Here's how the part is built. I have some questions about the finished solid (model axes, mm). Round coordinates to 2 decimals unless told otherwise and drop trailing zeros. Loops run counter-clockwise (first coordinate to the right, second up) from the corner with the lowest first, then second, coordinate; pieces in that order, holes last. Notation, with made-up numbers: (55, 81) - (101, 81) arc R25 ccw to (101, 114) - close; hole circle Ø5 at (-23.75, 13). An arc over 180 degrees is marked (long way). Return JSON: item names as keys, results as strings. Group by question number.
Autodesk Inventor part; units mm, degrees
ref_plane "YZ Plane" through (0, 0, 0) normal (1, 0, 0) x (0, 1, 0)
ref_plane "XZ Plane" through (0, 0, 0) normal (0, 1, 0) x (-1, 0, 0)
ref_plane "XY Plane" through (0, 0, 0) normal (0, 0, 1) x (1, 0, 0)
sketch "Sketch1" plane through (0, 0, 0) normal (0, 1, 0) x (-1, 0, 0)
  line L0 (0, 0) -> (400, 0)
  line L1 (400, 0) -> (400, -100)
  line L2 (400, -100) -> (0, -100)
  line L3 (320, -103) -> (320, -100)
  line L4 (80, -103) -> (80, -100)
  line L5 (240, -100) -> (240, -103)
  line L6 (160, -103) -> (160, -100)
  line L7 (400, -25) -> (400, -50)
  line L8 (200, 0) -> (200, -100) construction
  line L9 (320, -103) -> (240, -103)
  line L10 (160, -103) -> (80, -103)
  line L11 (400, 0) -> (0, 0)
  line L12 (400, -100) -> (400, 0)
  line L13 (400, -25) -> (400, -50)
  line L14 (400, 0) -> (400, -100)
  line L15 (0, -100) -> (0, 0)
  line L16 (403, -80) -> (400, -80)
  line L17 (403, -80) -> (403, -60)
  line L18 (403, -60) -> (400, -60)
  line L19 (403, -40) -> (400, -40)
  line L20 (403, -40) -> (403, -20)
  line L21 (403, -20) -> (400, -20)
  line L22 (0, -25) -> (0, -50)
  line L23 (0, -25) -> (0, -50)
  line L24 (0, -100) -> (0, 0)
  line L25 (-3, -80) -> (0, -80)
  line L26 (-3, -80) -> (-3, -60)
  line L27 (-3, -60) -> (0, -60)
  line L28 (-3, -40) -> (0, -40)
  line L29 (-3, -40) -> (-3, -20)
  line L30 (-3, -20) -> (0, -20)
  dimension "d1" = 100
  dimension "d7" = 3
  dimension "d8" = 80
  dimension "d17" = 20
  dimension "d18" = 20
  dimension "d19" = 20
extrude "Extrusion1" add sketch "Sketch1" along normal blind 3
properties part number "Estante int"
Q1. Imagine slicing it at A-A, the plane y = 1.35. List the corners of the cut face in (x, z) for me.
Q2. Will these pins go through, and if not, where does the flat tip stop? pin 1 Ø0.9 at (x, y) = (-353, 2) entering from -Z; pin 2 Ø0.9 at (y, z) = (2, -91.5) entering from -X; pin 3 Ø1.5 at (x, y) = (1.5, 2) entering from -Z.
Q3. Imagine slicing it at B-B, the plane x = -378. List the corners of the cut face in (y, z) for me.
Q4. Please list where these lines run through material, in increasing order: line 1 (X direction, y = 1.45, z = -91); line 2 (Z direction, x = -162.5, y = 0.9).
Output values:
{
 "1": {"outline": "(-403, -80) - (-400, -80) - (-400, -100) - (-320, -100) - (-320, -103) - (-240, -103) - (-240, -100) - (-160, -100) - (-160, -103) - (-80, -103) - (-80, -100) - (0, -100) - (0, -80) - (3, -80) - (3, -60) - (0, -60) - (0, -40) - (3, -40) - (3, -20) - (0, -20) - (0, 0) - (-400, 0) - (-400, -20) - (-403, -20) - (-403, -40) - (-400, -40) - (-400, -60) - (-403, -60) - close"},
 "2": {"pin 1": "stops at z = -100", "pin 2": "stops at x = -400", "pin 3": "stops at z = -80"},
 "3": {"outline": "(0, -100) - (3, -100) - (3, 0) - (0, 0) - close"},
 "4": {"line 1": "x = -400 to 0", "line 2": "z = -100 to 0"}
}
